For this review, take the finished solid that the model builds, in its own axes (mm). Face numbers are marked on the shaded views. A direction names the side the tool comes from. Round coordinates to 2 decimals unless told otherwise and drop trailing zeros. Write each loop counter-clockwise with the first axis right and the second up, starting at its lowest first coordinate (ties: lowest second). Pieces come first, ordered by that corner, then holes. Notation, with made-up numbers: (70.5, 31) -> (108.5, 31) arc R9 ccw to (108.5, 37) -> close; hole circle Ø1 at (89, 62.25). An arc over 180 degrees is marked (long way). Answer in a Markdown table with one row per item.
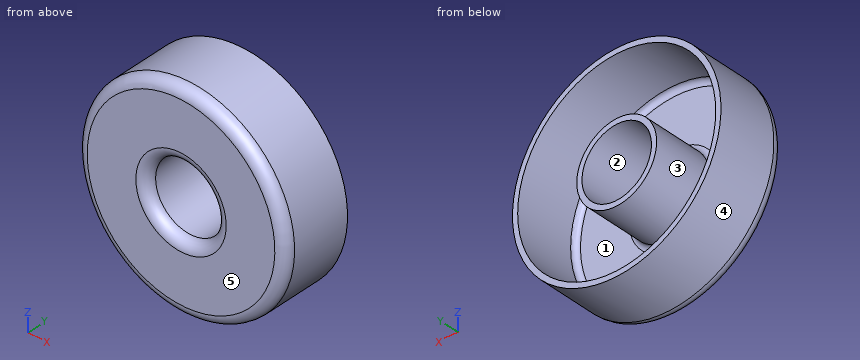
from build123d import *


with BuildPart() as part:
    # Sketch2 → Revolve1 (revolve)
    with BuildSketch(Plane(origin=(0, 0, 0), x_dir=(0, 0, -1), z_dir=(1, 0, 0))):
        with BuildLine():
            Line((-5, 4.25), (-5, -4.25))
            ThreePointArc((-5, -4.25), (-5.439339828, -5.310660172), (-6.5, -5.75))
            Line((-6.5, -5.75), (-13.5, -5.75))
            ThreePointArc((-13.5, -5.75), (-14.560660172, -5.310660172), (-15, -4.25))
            Line((-15, -4.25), (-15, 4.25))
            Line((-15, 4.25), (-14.25, 4.25))
            Line((-14.25, 4.25), (-14.25, -4.25))
            ThreePointArc((-14.25, -4.25), (-14.030330086, -4.780330086), (-13.5, -5))
            Line((-13.5, -5), (-6.5, -5))
            ThreePointArc((-6.5, -5), (-5.969669914, -4.780330086), (-5.75, -4.25))
            Line((-5.75, -4.25), (-5.75, 4.25))
            Line((-5.75, 4.25), (-5, 4.25))
        make_face()
    revolve(axis=Axis((0, 14.872392435, 0), (0, -1, 0)))


solid = part.part
1) Mouldability with a two-part tool opening along X and no side actions: class the marked faces 3, 4 and 5 as pulls with the +X half, pulls with the -X half, needs draft (parallel to the pull), parting line crosses it, or undercut.
Solved:
| item | result |
|---|---|
| face 3 | undercut |
| face 4 | parting line crosses it |
| face 5 | needs draft |
2) For line 1 (X direction, y = 1.25, z = 0); line 2 (Z direction, x = -1, y = -1), list the stretches that pass through material, from the lowest coordinate up. Write a range as [from, to].
Solved:
| item | result |
|---|---|
| line 1 | [-15, -14.25], [-5.75, -5], [5, 5.75], [14.25, 15] |
| line 2 | [-14.97, -14.21], [-5.66, -4.9], [4.9, 5.66], [14.21, 14.97] |
3) Consider section C-C on z = 0. State the section outline as (x, y) points.
Solved:
| item | result |
|---|---|
| outline | (-15, -4.25) arc R1.5 ccw to (-13.5, -5.75) -> (-6.5, -5.75) arc R1.5 ccw to (-5, -4.25) -> (-5, 4.25) -> (-5.75, 4.25) -> (-5.75, -4.25) arc R0.75 cw to (-6.5, -5) -> (-13.5, -5) arc R0.75 cw to (-14.25, -4.25) -> (-14.25, 4.25) -> (-15, 4.25) -> close; (5, -4.25) arc R1.5 ccw to (6.5, -5.75) -> (13.5, -5.75) arc R1.5 ccw to (15, -4.25) -> (15, 4.25) -> (14.25, 4.25) -> (14.25, -4.25) arc R0.75 cw to (13.5, -5) -> (6.5, -5) arc R0.75 cw to (5.75, -4.25) -> (5.75, 4.25) -> (5, 4.25) -> close |
4) For the marked faces 1 and 2, list the 3-axis set-ups (+Z, -Z, +X, -X, +Y, -Y) from which the entire face can be reached by the end or side of a thin tool; tool diameter is ignored.
Solved:
| item | result |
|---|---|
| face 1 | +Y |
| face 2 | +Y, -Y |
5) Consider section A-A on x = 0. State the section outline as (y, z) points.
Solved:
| item | result |
|---|---|
| outline | (-5.75, -13.5) arc R1.5 ccw to (-4.25, -15) -> (4.25, -15) -> (4.25, -14.25) -> (-4.25, -14.25) arc R0.75 cw to (-5, -13.5) -> (-5, -6.5) arc R0.75 cw to (-4.25, -5.75) -> (4.25, -5.75) -> (4.25, -5) -> (-4.25, -5) arc R1.5 ccw to (-5.75, -6.5) -> close; (-5.75, 6.5) arc R1.5 ccw to (-4.25, 5) -> (4.25, 5) -> (4.25, 5.75) -> (-4.25, 5.75) arc R0.75 cw to (-5, 6.5) -> (-5, 13.5) arc R0.75 cw to (-4.25, 14.25) -> (4.25, 14.25) -> (4.25, 15) -> (-4.25, 15) arc R1.5 ccw to (-5.75, 13.5) -> close |
6) Consider section B-B on y = -1.25. State the section outline as (x, z) points.
Solved:
| item | result |
|---|---|
| outline | circle Ø30 at (0, 0); circle Ø11.5 at (0, 0); hole circle Ø28.5 at (0, 0); hole circle Ø10 at (0, 0) |
7) Clearance check with flat-ended pins moving along their axes: pin 1 Ø1.5 at (x, z) = (-7.5, -10) entering from +Y; pin 2 Ø3 at (y, z) = (-4.5, -10) entering from -X; pin 3 Ø3 at (y, z) = (-4.5, -2.5) entering from +X; pin 4 Ø13.5 at (x, z) = (-1.5, 4) entering from +Y. State where each tip first meets the part, or that it passes through.
Solved:
| item | result |
|---|---|
| pin 1 | y = -5 |
| pin 2 | x = -12.35 |
| pin 3 | x = 14.97 |
| pin 4 | y = 4.25 |
